from build123d import *

# Parameters (mm, degrees)
SKETCH1_R           = 5
SKETCH1_R_2         = 1.55
SKETCH1_W           = 20
SKETCH1_H           = 3
SKETCH1_W_2         = 9
SKETCH1_H_2         = 9
BOSS_EXTRUDE1_DEPTH = 1.5


with BuildPart() as part:
    # Sketch1 → Boss-Extrude1 (new body, symmetric)
    with BuildSketch(Plane(origin=(0, 0, 0), x_dir=(1, 0, 0), z_dir=(0, 1, 0))):
        with BuildLine():
            Line((0, 15), (185, 15))
            ThreePointArc((185, 15), (200, 0), (185, -15))
            Line((185, -15), (0, -15))
            ThreePointArc((0, -15), (-15, 0), (0, 15))
        make_face()
        Circle(SKETCH1_R, mode=Mode.SUBTRACT)
        with Locations((5.051814855, 8.75)):
            Circle(SKETCH1_R_2, mode=Mode.SUBTRACT)
        with Locations((10.103629711, 0)):
            Circle(SKETCH1_R_2, mode=Mode.SUBTRACT)
        with Locations((5.051814855, -8.75)):
            Circle(SKETCH1_R_2, mode=Mode.SUBTRACT)
        with Locations((-5.051814855, -8.75)):
            Circle(SKETCH1_R_2, mode=Mode.SUBTRACT)
        with Locations((-10.103629711, 0)):
            Circle(SKETCH1_R_2, mode=Mode.SUBTRACT)
        with Locations((-5.051814855, 8.75)):
            Circle(SKETCH1_R_2, mode=Mode.SUBTRACT)
        with Locations((92.5, 0)):
            Rectangle(SKETCH1_W, SKETCH1_H, mode=Mode.SUBTRACT)
        with Locations((185, 0)):
            Rectangle(SKETCH1_W_2, SKETCH1_H_2, mode=Mode.SUBTRACT)
    extrude(amount=BOSS_EXTRUDE1_DEPTH, both=True)


solid = part.part
Here's how the part is built. I have some questions about the finished solid (model axes, mm). Round coordinates to 2 decimals unless told otherwise and drop trailing zeros. One line per question, with ' | ' between items.
1) I need wall thicknesses on line 1 (X direction, y = 1.1, z = 3); line 2 (X direction, y = -0.6, z = 0); line 3 (X direction, y = 0.95, z = -9). Which ranges of each line are inside material? Lowest first, please.
Checked values:
line 1: x = -14.7 to -4, 4 to 180.5, 189.5 to 199.7 | line 2: x = -15 to -11.65, -8.55 to -5, 5 to 8.55, 11.65 to 82.5, 102.5 to 180.5, 189.5 to 200 | line 3: x = -12 to -6.58, -3.52 to 3.52, 6.58 to 197
2) We'd pull the mould along Z, two halves only. Please class faces 1 (the cylindrical face through (-15, 0, 0)), 2 (the flat face through (94, -1.5, -4)), 3 (the cylindrical face through (-1.08, -0.02, 4.88)): released by +Z, released by -Z, zero draft, split by the parting line, or undercut.
Checked values:
face 1: split by the parting line | face 2: zero draft | face 3: undercut
3) I'm going to push flat-ended pins straight in: pin 1 Ø4 at (x, z) = (-10.1, 0) entering from -Y; pin 2 Ø2.5 at (x, z) = (5.05, 8.75) entering from +Y (1 decimal); pin 3 Ø1.5 at (y, z) = (-1, 11) entering from +X; pin 4 Ø1.5 at (x, y) = (186.5, -0.5) entering from +Z. Where does each tip first touch, or does it pass through?
Checked values:
pin 1: stops at y = -1.5 | pin 2: passes through | pin 3: stops at x = 195.95 | pin 4: stops at z = 14.98
4) Imagine slicing it at A-A, the plane y = 0.1. Count the separate pieces of the cut face and the enclosed holes in it, plus the area to 3 significant figures.
Checked values:
separate pieces: 1 | enclosed holes: 9 | area: 5,990 mm²
